from build123d import *

# Parameters (mm, degrees)
SKETCH_1_R      = 1.5
EXTRUDE_1_DEPTH = 13.5
SKETCH_2_R      = 1
EXTRUDE_2_DEPTH = 3
SKETCH_3_R      = 1
EXTRUDE_3_DEPTH = 3
SKETCH_4_R      = 1.5
EXTRUDE_4_DEPTH = 1


with BuildPart() as part:
    # 草图1 → 凸台-拉伸1 (new body)
    with BuildSketch(Plane.XY):
        Circle(SKETCH_1_R)
    extrude(amount=EXTRUDE_1_DEPTH)

    # 草图2 → 凸台-拉伸2 (add)
    with BuildSketch(Plane.XY.offset(13.5)):
        Circle(SKETCH_2_R)
    extrude(amount=EXTRUDE_2_DEPTH)

    # 草图3 → 凸台-拉伸3 (add)
    with BuildSketch(Plane(origin=(0, 0, 0), x_dir=(-1, 0, 0), z_dir=(0, 0, -1))):
        Circle(SKETCH_3_R)
    extrude(amount=EXTRUDE_3_DEPTH)

    # 草图4 → 凸台-拉伸4 (add)
    with BuildSketch(Plane(origin=(0, 0, -3), x_dir=(-1, 0, 0), z_dir=(0, 0, -1))):
        Circle(SKETCH_4_R)
    extrude(amount=EXTRUDE_4_DEPTH)


solid = part.part
Part model, mm, in its own coordinate system. A direction names the side the tool comes from. Coordinates: 2 decimals unless noted, no trailing zeros. Loops run counter-clockwise (first coordinate to the right, second up) from the corner with the lowest first, then second, coordinate; pieces in that order, holes last. Notation, with made-up numbers: (48.5, 8.5) - (58.5, 8.5) arc R21 cw to (58.5, 38.5) - close; hole circle Ø9 at (49, 55.25). An arc over 180 degrees is marked (long way). Write each question's results on one line, items separated by ' | '. Start each with the question number.
Q1. Which spindle directions (+Z, -Z, +X, -X, +Y, -Y) get a long thin tool onto all of the face, cutting with end or side? Do faces 1 (the cylindrical face through (-1.5, 0.07, 6.66)), 2 (the cylindrical face through (0, -1, 15)). Say none if no direction does.
Q2. Probe line 1 along Z through (x, y) = (0.6, 1.25); line 2 along Y through (x, z) = (-0.9, 15); line 3 along Y through (x, z) = (0.85, 13.25). List the from-to ranges inside material, lowest first.
Q3. Slice it at A-A on x = -1.2. Give the cut face in (y, z), and give its area (3 significant figures).
Q4. Two-plate mould, pull along Z, no slides. Class faces 3 (the flat face through (0, 0, -4)), 4 (the cylindrical face through (0, -1, -1)), 5 (the flat face through (0, 0, 16.5)): +Z half, -Z half, draft (parallel to the pull), parting line (faces both ways), or undercut.
Q5. Slice it at D-D on z = 0.75. Give the cut face in (x, y).
Q6. Slice it at B-B on x = 0. Give the cut face in (y, z).
Answer:
1) face 1: +Z, -Z | face 2: +Z
2) line 1: z = -4 to -3, 0 to 13.5 | line 2: y = -0.44 to 0.44 | line 3: y = -1.24 to 1.24
3) outline: (-0.9, -4) - (0.9, -4) - (0.9, -3) - (-0.9, -3) - close; (-0.9, 0) - (0.9, 0) - (0.9, 13.5) - (-0.9, 13.5) - close | area: 26.1 mm2
4) face 3: -Z half | face 4: undercut | face 5: +Z half
5) outline: circle Ø3 at (0, 0)
6) outline: (-1.5, -4) - (1.5, -4) - (1.5, -3) - (1, -3) - (1, 0) - (1.5, 0) - (1.5, 13.5) - (1, 13.5) - (1, 16.5) - (-1, 16.5) - (-1, 13.5) - (-1.5, 13.5) - (-1.5, 0) - (-1, 0) - (-1, -3) - (-1.5, -3) - close
